Part model, mm, in its own coordinate system. A direction names the side the tool comes from. Round coordinates to 2 decimals unless told otherwise and drop trailing zeros. Loops run counter-clockwise (first coordinate to the right, second up) from the corner with the lowest first, then second, coordinate; pieces in that order, holes last.
(1) Cut at D-D on y = -2. Count the separate pieces of the cut face and the enclosed holes in it, then the cut area to 3 significant figures.
(2) Probe probe 1 along Z at (x, y) = (0, -5.75) (3 decimals); probe 2 along Y at (x, z) = (1.75, 0); probe 3 along Y at (x, z) = (-6.5, -2.75). List the from-to ranges inside material, lowest first.
(3) Flat gauge pins, fed straight in: pin 1 (0.6 mm diameter, centred on x = 0.5, z = -3.5, fed in from -Y); pin 2 (4 mm diameter, centred on x = 6, y = 14, fed in from +Z); pin 3 (10 mm diameter, centred on y = -12, z = 6, fed in from -X). Where does each tip first touch, or does it go through?
(4) Tool access for faces 1 (the face through (0, 0, 0)), 2 (the face through (-4.747, 18.736, 4.733)): list every direction of +Z, -Z, +X, -X, +Y, -Y with a clear straight run to the whole face (end or side of a thin tool).
(5) Cut at C-C on z = 0. List the corners of the cut face in (x, y) (3 decimals), then the cut area to 3 significant figures.
(6) Cut at B-B on y = 7. List the corners of the cut face in (x, z) (3 decimals), then the cut area to 3 significant figures.
(7) Mould opens along Z. For faces 3 (the face through (-6, 19.05, 0)), 4 (the face through (0, 13, -4.826)), 5 (the face through (-0.34, -1.63, 2.42)) say: +Z half, -Z half, draft (parallel to the pull), parting line (faces both ways), or undercut.
from build123d import *

# Parameters (mm, degrees)
F0_R     = 1.5875
F1_DEPTH = 3.81
F2_R     = 9.525
F2_R_2   = 8.0221390402
F3_DEPTH = 19.05
F4_R     = 9.525
F5_DEPTH = 19.05
F6_W     = 9.652
F6_H     = 9.652
F7_DEPTH = 12.7
F8_R     = 0.762
F9_SIZE  = 0.508


with BuildPart() as f1:
    # F0 (on Front) → F1 (new body)
    with BuildSketch(Plane.XZ):
        with Locations((0, 3.96875)):
            Circle(F0_R)
    extrude(amount=F1_DEPTH)



with BuildPart() as f1b:
    # F0 (on Front) → F1, piece 2 (new body)
    with BuildSketch(Plane.XZ):
        with Locations((0, -3.96875)):
            Circle(F0_R)
    extrude(amount=F1_DEPTH)


with BuildPart() as f3:
    # F2 (on face) → F3 (new body)
    with BuildSketch(Plane.XZ):
        Circle(F2_R)
        Circle(F2_R_2, mode=Mode.SUBTRACT)
    extrude(amount=F3_DEPTH)


with BuildPart() as f1_1:
    add(f1.part)

    add(f1b.part)  # F5 merges F1b

    add(f3.part)  # F5 merges F3
    # F4 (on face) → F5 (join)
    with BuildSketch(Plane(origin=(0, 0, 0), x_dir=(-1, 0, 0), z_dir=(0, 1, 0))):
        Circle(F4_R)
    extrude(amount=F5_DEPTH)

    # F6 (on face) → F7 (cut)
    with BuildSketch(Plane(origin=(0, 19.05, 0), x_dir=(-1, 0, 0), z_dir=(0, 1, 0))):
        Rectangle(F6_W, F6_H)
    extrude(amount=-F7_DEPTH, mode=Mode.SUBTRACT)

    # F8
    f8_edges = [f1_1.edges().sort_by_distance(p)[0] for p in [
        (-4.826, 12.7, -4.826),
        (-4.826, 12.7, 4.826),
        (4.826, 12.7, 4.826),
        (4.826, 12.7, -4.826),
    ]]
    fillet(f8_edges, radius=F8_R)

    # F9
    f9_edges = [f1_1.edges().sort_by_distance(p)[0] for p in [
        (0, 19.05, -4.826),
        (9.525, 19.05, 0),
        (-9.525, -19.05, 0),
        (-8.022139, -19.05, 0),
        (-1.5875, -3.81, 3.96875),
        (-1.5875, -3.81, -3.96875),
    ]]
    chamfer(f9_edges, length=F9_SIZE)


solid = f1_1.part
Final values:
1. separate pieces: 3
1. enclosed holes: 1
1. area: 98.7 mm2
2. probe 1: z = -9.525 to -8.022, 8.022 to 9.525
2. probe 2: y = 0 to 6.35
2. probe 3: y = 0 to 19.05
3. pin 1: stops at y = -3.81
3. pin 2: stops at z = 8.64
3. pin 3: stops at x = -9.47
4. face 1: -Y
4. face 2: +Y
5. outline: (-9.525, -18.542) - (-9.017, -19.05) - (-8.53, -19.05) - (-8.022, -18.542) - (-8.022, 0) - (8.022, 0) - (8.022, -18.542) - (8.53, -19.05) - (9.017, -19.05) - (9.525, -18.542) - (9.525, 18.542) - (9.017, 19.05) - (5.334, 19.05) - (4.826, 18.542) - (4.826, 6.35) - (-4.826, 6.35) - (-4.826, 18.542) - (-5.334, 19.05) - (-9.017, 19.05) - (-9.525, 18.542) - close
5. area: 297 mm2
6. outline: circle Ø19.05 at (0, 0); hole (-4.826, -4.064) arc R0.762 ccw to (-4.064, -4.826) - (4.064, -4.826) arc R0.762 ccw to (4.826, -4.064) - (4.826, 4.064) arc R0.762 ccw to (4.064, 4.826) - (-4.064, 4.826) arc R0.762 ccw to (-4.826, 4.064) - close
6. area: 192 mm2
7. face 3: draft
7. face 4: undercut
7. face 5: undercut
